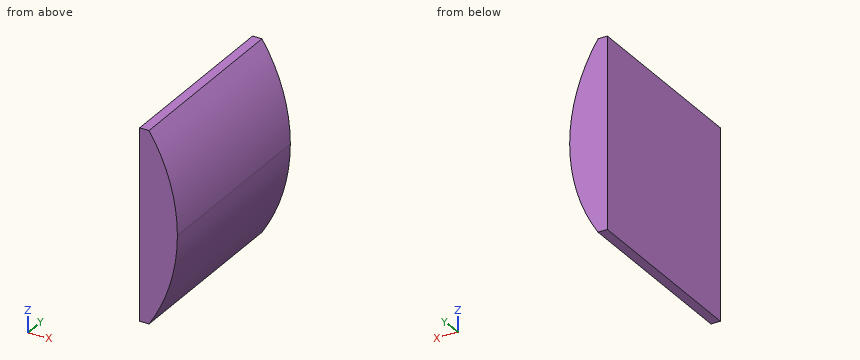
```python
from build123d import *

# Parameters (mm, degrees)
EXTRUDE_1_DEPTH = 20
SKETCH_2_W      = 20.253995302
SKETCH_2_H      = 20
EXTRUDE_2_DEPTH = 1


with BuildPart() as part:
    # 草图1 → 凸台-拉伸1 (new body)
    with BuildSketch(Plane(origin=(0, 0, 0), x_dir=(1, 0, 0), z_dir=(0, 1, 0))):
        with BuildLine():
            ThreePointArc((1.545950546, 0), (0.774439181, 5.28408774), (-1.475680066, 10.126997651))
            Line((-1.475680066, 10.126997651), (-1.475680066, -10.126997651))
            ThreePointArc((-1.475680066, -10.126997651), (0.774439181, -5.28408774), (1.545950546, 0))
        make_face()
    extrude(amount=EXTRUDE_1_DEPTH)

    # 草图2 → 凸台-拉伸2 (add)
    with BuildSketch(Plane.ZY.offset(1.475680066)):
        with Locations((0, 10)):
            Rectangle(SKETCH_2_W, SKETCH_2_H)
    extrude(amount=EXTRUDE_2_DEPTH)


solid = part.part
```
Check sheet for the modelled part. Datum: model origin and axes. Units: mm. Give positions to 0.01 mm unless a question says otherwise; leave off trailing zeros. Order: outer loops, then holes, each group sorted by start corner. A loop starts at its lowest first (then second) coordinate and runs counter-clockwise, first axis right, second up. Notation, with made-up numbers: (-32.5, 26) -> (-16.5, 26) arc R25 ccw to (-16.5, 41) -> close; hole circle Ø7 at (51, 80). An arc over 180 degrees is marked (long way). Use CSV: the item, a comma, the result in double quotes. Start each with the question number.
1) Go/stop test with flat-tipped pins: P1, Ø5, axis at y = 17.5, z = 4, coming from the +X side (3 decimals); P2, Ø1.5, axis at x = 0, y = 6, coming from the +Z side; P3, Ø1.5, axis at x = 0.5, y = 13.5, coming from the +Z side. Record where each tip stops, or that it passes through.
2) Sectioned sample at A-A, the plane y = 17. Record the boundary of the cut face in (x, z).
3) Sectioned sample at B-B, the plane x = 0.75. Record the boundary of the cut face in (y, z).
4) Material ranges on line 1 (X direction, y = 17, z = -1.75); line 2 (X direction, y = 2, z = -5.5); line 3 (Z direction, x = -0.65, y = 2.5), recorded low to high. Write a range as from..to.
5) Sectioned sample at C-C, the plane z = -4.75. Record the boundary of the cut face in (x, y), plus the area to 3 significant figures.
Recorded:
1,P1,"x = 1.485"
1,P2,"z = 8.92"
1,P3,"z = 7.95"
2,outline,"(-2.48, -10.13) -> (-1.48, -10.13) arc R18.48 ccw to (-1.48, 10.13) -> (-2.48, 10.13) -> close"
3,outline,"(0, -5.37) -> (20, -5.37) -> (20, 5.37) -> (0, 5.37) -> close"
4,line 1,"-2.48..1.46"
4,line 2,"-2.48..0.71"
4,line 3,"-8.74..8.74"
5,outline,"(-2.48, 0) -> (0.93, 0) -> (0.93, 20) -> (-2.48, 20) -> close"
5,area,"68.0 mm2"
